Can you work these out from the model? Positions are in its coordinate system, mm. Face numbers are marked on the shaded views. A direction names the side the tool comes from. Round coordinates to 2 decimals unless told otherwise and drop trailing zeros. Loops run counter-clockwise (first coordinate to the right, second up) from the corner with the lowest first, then second, coordinate; pieces in that order, holes last. Notation, with made-up numbers: (35, 47) -> (79, 47) arc R18 cw to (79, 73) -> close; hole circle Ø1 at (83, 49). An arc over 180 degrees is marked (long way). Answer as a JSON object with one key per item and string values.
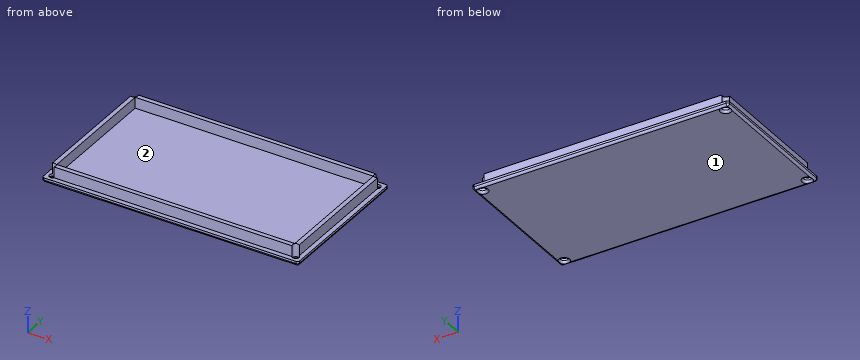
```python
from build123d import *

# Parameters (mm, degrees)
BOSS_EXTRUDE1_DEPTH                        = 2
SKETCH2_W                                  = 113.60000000000001
SKETCH2_H                                  = 62.1
SKETCH2_W_2                                = 109.60000000000001
SKETCH2_H_2                                = 58.1
BOSS_EXTRUDE2_DEPTH                        = 5
SKETCH3_R                                  = 1.5000000000000042
CUT_EXTRUDE2_DEPTH                         = 71.85433681838424
MIRROR3_AT_THE_SECOND_PLANE_COPY_1_SKETC_R = 1.5000000000000042
MIRROR3_AT_THE_SECOND_PLANE_COPY_1_DEPTH   = 71.85433681838424
FILLET1_R                                  = 1
FILLET2_R                                  = 1


with BuildPart() as part:
    # Sketch1 → Boss-Extrude1 (new body)
    with BuildSketch(Plane.XY):
        Polygon((-55.697933748362985, 33.2), (62.20206625163701, 33.2), (62.202066251637014, -33.2), (-55.697933748362985, -33.2), align=None)
    extrude(amount=BOSS_EXTRUDE1_DEPTH)

    # Sketch2 → Boss-Extrude2 (add)
    with BuildSketch(Plane.XY.offset(2)):
        with Locations((3.252066251637011, 0)):
            Rectangle(SKETCH2_W, SKETCH2_H)
        with Locations((3.252066251637011, 0)):
            Rectangle(SKETCH2_W_2, SKETCH2_H_2, mode=Mode.SUBTRACT)
    extrude(amount=BOSS_EXTRUDE2_DEPTH)

    # Sketch3 → Cut-Extrude2 (cut, symmetric)
    with BuildSketch(Plane(origin=(0, 0, 0), x_dir=(-1, 0, 0), z_dir=(0, 0, -1))):
        with Locations(Location((-59.202066251637, 30.200000000000003, 0), (0, 0, 34.518107841))):
            Circle(SKETCH3_R)
    cut_extrude2 = extrude(amount=CUT_EXTRUDE2_DEPTH, both=True, mode=Mode.SUBTRACT)

    # Mirror2: Cut-Extrude2 across plane
    add(cut_extrude2.mirror(Plane.ZX), mode=Mode.SUBTRACT)

    # Mirror3: Cut-Extrude2 across plane
    add(cut_extrude2.mirror(Plane.ZX), mode=Mode.SUBTRACT)

    # Mirror3 at the second plane: Cut-Extrude2 across plane
    add(cut_extrude2.mirror(Plane(origin=(3.2520662516370114, 0, 0), x_dir=(0, 0, 1), z_dir=(1, 0, 0))), mode=Mode.SUBTRACT)

    # Mirror3 at the second plane copy 1 sketc → Mirror3 at the second plane copy 1 (cut, symmetric)
    with BuildSketch(Plane(origin=(6.504132503274023, 0, 0), x_dir=(1, 0, 0), z_dir=(0, 0, -1))):
        with Locations(Location((-59.202066251637, 30.200000000000003, 0), (0, 0, 34.518107841))):
            Circle(MIRROR3_AT_THE_SECOND_PLANE_COPY_1_SKETC_R)
    extrude(amount=MIRROR3_AT_THE_SECOND_PLANE_COPY_1_DEPTH, both=True, mode=Mode.SUBTRACT)

    # Fillet1
    fillet1_edges = [part.edges().sort_by_distance(p)[0] for p in [
        (62.202066251637014, -33.2, 1),
        (-55.697933748362985, -33.2, 1),
        (-55.697933748362985, 33.2, 1),
        (62.20206625163701, 33.2, 1),
    ]]
    fillet(fillet1_edges, radius=FILLET1_R)

    # Fillet2
    # the kernel refuses this fillet: 1 mm, written as the material it takes off along each edge
    with BuildSketch(Plane(origin=(62.20206625163701, 32.2, 0), x_dir=(-1, -1.1e-16, 0), z_dir=(1.1e-16, -1, 0)), Plane(origin=(-55.697933748362985, -32.2, 0), x_dir=(1, 0, 0), z_dir=(0, 1, 0))) as fillet2_piece_1:
        with BuildLine():
            CenterArc((FILLET2_R, -FILLET2_R), FILLET2_R, 90, 90)
            Line((0, -FILLET2_R), (0, 0))
            Line((0, 0), (FILLET2_R, 0))
        make_face()
    extrude(amount=64.4, mode=Mode.SUBTRACT)
    with BuildSketch(Plane(origin=(61.202066251637014, -33.2, 0), x_dir=(0, 1, 0), z_dir=(-1, 0, 0))) as fillet2_piece_2:
        with BuildLine():
            CenterArc((FILLET2_R, -FILLET2_R), FILLET2_R, 90, 90)
            Line((0, -FILLET2_R), (0, 0))
            Line((0, 0), (FILLET2_R, 0))
        make_face()
    extrude(amount=115.9, mode=Mode.SUBTRACT)
    with BuildSketch(Plane(origin=(-54.697933748362985, 33.2, 0), x_dir=(0, 0, 1), z_dir=(1, 0, 0))) as fillet2_piece_3:
        with BuildLine():
            CenterArc((FILLET2_R, FILLET2_R), FILLET2_R, 180, 90)
            Line((-1.1e-16, FILLET2_R), (0, 0))
            Line((0, 0), (FILLET2_R, 0))
        make_face()
    extrude(amount=115.89999999999999, mode=Mode.SUBTRACT)
    with BuildSketch(Plane(origin=(-54.697933748362985, -32.2, 0), x_dir=(-1, 0, 0), z_dir=(0, 1, 0))) as fillet2_piece_4:
        with BuildLine():
            CenterArc((1 - FILLET2_R, FILLET2_R), FILLET2_R, 270, 90)
            Line((1, FILLET2_R), (1, 0))
            Line((1, 0), (1 - FILLET2_R, 0))
        make_face()
    revolve(axis=Axis((-54.697933748362985, -32.2, 0), (0, 0, 1)), revolution_arc=90, mode=Mode.SUBTRACT)
    with BuildSketch(Plane(origin=(-54.697933748362985, 32.2, 0), x_dir=(0, 1, 0), z_dir=(1, 0, 0))) as fillet2_piece_5:
        with BuildLine():
            CenterArc((1 - FILLET2_R, FILLET2_R), FILLET2_R, 270, 90)
            Line((1, FILLET2_R), (1, 0))
            Line((1, 0), (1 - FILLET2_R, 0))
        make_face()
    revolve(axis=Axis((-54.697933748362985, 32.2, 0), (0, 0, 1)), revolution_arc=90, mode=Mode.SUBTRACT)
    with BuildSketch(Plane(origin=(61.20206625163701, 32.2, 0), x_dir=(0, 1, 0), z_dir=(-1, 0, 0))) as fillet2_piece_6:
        with BuildLine():
            CenterArc((1 - FILLET2_R, -FILLET2_R), FILLET2_R, 6.36e-15, 90)
            Line((1, -FILLET2_R), (1, 0))
            Line((1, 0), (1 - FILLET2_R, 0))
        make_face()
    revolve(axis=Axis((61.20206625163701, 32.2, 0), (0, 0, -1)), revolution_arc=90, mode=Mode.SUBTRACT)
    with BuildSketch(Plane(origin=(61.202066251637014, -32.2, 0), x_dir=(1, 0, 0), z_dir=(0, 1, 0))) as fillet2_piece_7:
        with BuildLine():
            CenterArc((1 - FILLET2_R, -FILLET2_R), FILLET2_R, 6.36e-15, 90)
            Line((1, -FILLET2_R), (1, 0))
            Line((1, 0), (1 - FILLET2_R, 0))
        make_face()
    revolve(axis=Axis((61.202066251637014, -32.2, 0), (0, 0, -1)), revolution_arc=90, mode=Mode.SUBTRACT)
    with BuildSketch(Plane(origin=(59.202066251637, 30.200000000000003, 0), x_dir=(-0.8239471396211576, 0.5666666666657856, 0), z_dir=(-0.5666666666657856, -0.8239471396211576, 0))) as fillet2_piece_8:
        with BuildLine():
            CenterArc((1.5000000000000024 + FILLET2_R, -FILLET2_R), FILLET2_R, 90, 90)
            Line((1.5000000000000024, -FILLET2_R), (1.5000000000000024, 0))
            Line((1.5000000000000024, 0), (1.5000000000000024 + FILLET2_R, 0))
        make_face()
    revolve(axis=Axis((59.202066251637, 30.200000000000003, 0), (0, 0, -1)), mode=Mode.SUBTRACT)
    with BuildSketch(Plane(origin=(59.202066251637, -30.200000000000003, 0), x_dir=(-0.8239471396211576, -0.5666666666657856, 0), z_dir=(0.5666666666657856, -0.8239471396211576, 0))) as fillet2_piece_9:
        with BuildLine():
            CenterArc((1.5000000000000024 + FILLET2_R, -FILLET2_R), FILLET2_R, 90, 90)
            Line((1.5000000000000024, -FILLET2_R), (1.5000000000000024, 0))
            Line((1.5000000000000024, 0), (1.5000000000000024 + FILLET2_R, 0))
        make_face()
    revolve(axis=Axis((59.202066251637, -30.200000000000003, 0), (0, 0, -1)), mode=Mode.SUBTRACT)
    with BuildSketch(Plane(origin=(-52.69793374836298, 30.200000000000003, 0), x_dir=(0.8239471396211576, 0.5666666666657856, 0), z_dir=(-0.5666666666657856, 0.8239471396211576, 0))) as fillet2_piece_10:
        with BuildLine():
            CenterArc((1.5000000000000024 + FILLET2_R, -FILLET2_R), FILLET2_R, 90, 90)
            Line((1.5000000000000062, -FILLET2_R), (1.5000000000000024, 0))
            Line((1.5000000000000024, 0), (1.5000000000000024 + FILLET2_R, 0))
        make_face()
    revolve(axis=Axis((-52.69793374836298, 30.200000000000003, 0), (0, 0, -1)), mode=Mode.SUBTRACT)
    with BuildSketch(Plane(origin=(-52.69793374836298, -30.200000000000003, 0), x_dir=(0.8239471396211576, -0.5666666666657856, 0), z_dir=(0.5666666666657856, 0.8239471396211576, 0))) as fillet2_piece_11:
        with BuildLine():
            CenterArc((1.5000000000000024 + FILLET2_R, -FILLET2_R), FILLET2_R, 90, 90)
            Line((1.5000000000000062, -FILLET2_R), (1.5000000000000024, 0))
            Line((1.5000000000000024, 0), (1.5000000000000024 + FILLET2_R, 0))
        make_face()
    revolve(axis=Axis((-52.69793374836298, -30.200000000000003, 0), (0, 0, -1)), mode=Mode.SUBTRACT)


solid = part.part
```
Q1. I want a section at B-B, the plane x = -22. Write out the boundary of the cut face in (y, z).
Determined:
{"outline": "(-33.2, 1) arc R1 ccw to (-32.2, 0) -> (32.2, 0) arc R1 ccw to (33.2, 1) -> (33.2, 2) -> (31.05, 2) -> (31.05, 7) -> (29.05, 7) -> (29.05, 2) -> (-29.05, 2) -> (-29.05, 7) -> (-31.05, 7) -> (-31.05, 2) -> (-33.2, 2) -> close"}
Q2. I want a section at A-A, the plane z = 4.5. Write out the boundary of the cut face in (x, y), then the cut area to 3 significant figures.
Determined:
{"outline": "(-53.55, -28.96) arc R1.5 cw to (-51.46, -31.05) -> (57.97, -31.05) arc R1.5 cw to (60.05, -28.96) -> (60.05, 28.96) arc R1.5 cw to (57.97, 31.05) -> (-51.46, 31.05) arc R1.5 cw to (-53.55, 28.96) -> close; hole (-51.55, -29.05) -> (58.05, -29.05) -> (58.05, 29.05) -> (-51.55, 29.05) -> close", "area": "667 mm²"}
Q3. On a 3-axis mill with a long thin cutter (end or side, diameter ignored), from which of +Z, -Z, +X, -X, +Y, -Y can I reach the whole of each face in a straight line? I mean the marked faces 1 and 2. Say none if no direction works.
Determined:
{"face 1": "-Z, +X, -X, +Y, -Y", "face 2": "+Z"}
Q4. I'm going to push flat-ended pins straight in: pin 1 (2.5 mm diameter, centred on x = -15.5, z = 5, fed in from +Y); pin 2 (1 mm diameter, centred on x = 24.5, y = 22.5, fed in from -Z); pin 3 (4 mm diameter, centred on x = 59.2, y = 30.2, fed in from -Z); pin 4 (2.5 mm diameter, centred on y = -0.5, z = 4, fed in from +X). Where does each tip first touch, or does it pass through?
Determined:
{"pin 1": "y = 31.05", "pin 2": "z = 0", "pin 3": "z = 0.13", "pin 4": "x = 60.05"}
Q5. I want a section at C-C, the plane y = -20. Write out the boundary of the cut face in (x, z), then the cut area to 3 significant figures.
Determined:
{"outline": "(-55.7, 1) arc R1 ccw to (-54.7, 0) -> (61.2, 0) arc R1 ccw to (62.2, 1) -> (62.2, 2) -> (60.05, 2) -> (60.05, 7) -> (58.05, 7) -> (58.05, 2) -> (-51.55, 2) -> (-51.55, 7) -> (-53.55, 7) -> (-53.55, 2) -> (-55.7, 2) -> close", "area": "255 mm²"}
Q6. If I drill on L1, parallel to Y at x = 16, z = 2.5; L2, parallel to X at y = 10, z = 3.75; L3, parallel to Z at x = 57, y = 1, over which ranges is the centre line in solid material (lowest first)? Write a range as [from, to].
Determined:
{"L1": "[-31.05, -29.05], [29.05, 31.05]", "L2": "[-53.55, -51.55], [58.05, 60.05]", "L3": "[0, 2]"}
